from build123d import *

# Parameters (mm, degrees)
F0_R     = 4.5
F1_DEPTH = 10


with BuildPart() as f1:
    # F0 (on Top) → F1 (new body)
    with BuildSketch(Plane.XY):
        Polygon((-243.172072, 141.001241), (-243.172072, -226.998759), (-67.646502, -226.998759), (-67.646502, -191.498759), (-213.172072, -191.498759), (-213.172072, 105.501241), (-113.172072, 105.501241), (-113.172072, 141.001241), align=None)
        with Locations((-228.172072, -211.998759)):
            Circle(F0_R, mode=Mode.SUBTRACT)
        with Locations((-228.172072, 126.001241)):
            Circle(F0_R, mode=Mode.SUBTRACT)
        Polygon((-67.646502, -191.498759), (-67.646502, -226.998759), (16.827928, -226.998759), (16.827928, 141.001241), (-113.172072, 141.001241), (-113.172072, 105.501241), (-13.172072, 105.501241), (-13.172072, -191.498759), align=None)
        with Locations((1.827928, -211.998759)):
            Circle(F0_R, mode=Mode.SUBTRACT)
        with Locations((1.827928, 126.001241)):
            Circle(F0_R, mode=Mode.SUBTRACT)
    extrude(amount=F1_DEPTH)


solid = f1.part
The model under review builds one solid part; all positions refer to its coordinate system, in mm. A direction names the side the tool comes from. Round coordinates to 2 decimals unless told otherwise and drop trailing zeros. Loops run counter-clockwise (first coordinate to the right, second up) from the corner with the lowest first, then second, coordinate; pieces in that order, holes last. Notation, with made-up numbers: (-19, 47) - (19, 47) arc R16 ccw to (19, 58) - close; hole circle Ø10 at (89.5, 88). An arc over 180 degrees is marked (long way). Use CSV: the item, a comma, the result in double quotes.
(1) For line 1 (X direction, y = -14, z = 8.75); line 2 (Y direction, x = -64, z = 5.5), list the stretches that pass through material, from the lowest coordinate up.
Working result:
line 1,"x = -243.17 to -213.17, -13.17 to 16.83"
line 2,"y = -227 to -191.5, 105.5 to 141"
(2) Take a section at B-B, the plane y = -125. Give the boundary of the cut face in (x, z), plus the area to 3 significant figures.
Working result:
outline,"(-243.17, 0) - (-213.17, 0) - (-213.17, 10) - (-243.17, 10) - close; (-13.17, 0) - (16.83, 0) - (16.83, 10) - (-13.17, 10) - close"
area,"600 mm^2"
(3) Take a section at C-C, the plane z = 1.5. Give the boundary of the cut face in (x, y).
Working result:
outline,"(-243.17, -227) - (16.83, -227) - (16.83, 141) - (-243.17, 141) - close; hole circle Ø9 at (-228.17, -212); hole circle Ø9 at (-228.17, 126); hole (-213.17, -191.5) - (-13.17, -191.5) - (-13.17, 105.5) - (-213.17, 105.5) - close; hole circle Ø9 at (1.83, -212); hole circle Ø9 at (1.83, 126)"
(4) Machinability: for faces 5 (the flat face through (-112, -191.499, 5)), 6 (the flat face through (1, -40, 0)), which of the approach directions +Z, -Z, +X, -X, +Y, -Y give a long, thin tool a straight path to every point of the face, cutting with its end or side? Answer none if there is none.
Working result:
face 5,"+Z, -Z"
face 6,"-Z, +X, -X, +Y, -Y"
(5) Take a section at A-A, the plane x = -65. Give the boundary of the cut face in (y, z), plus the area to 3 significant figures.
Working result:
outline,"(-227, 0) - (-191.5, 0) - (-191.5, 10) - (-227, 10) - close; (105.5, 0) - (141, 0) - (141, 10) - (105.5, 10) - close"
area,"710 mm^2"
(6) The part is to be moulded in two halves that separate along X. For faces 1 (the flat face through (-13.172, -41, 5)), 2 (the flat face through (-115, 105.501, 5)), 3 (the flat face through (-115, -226.999, 5)), 4 (the flat face through (16.828, -46, 5)), say which applies: pulls with the +X half, pulls with the -X half, needs draft (parallel to the pull), parting line crosses it, or undercut.
Working result:
face 1,"undercut"
face 2,"undercut"
face 3,"needs draft"
face 4,"pulls with the +X half"
